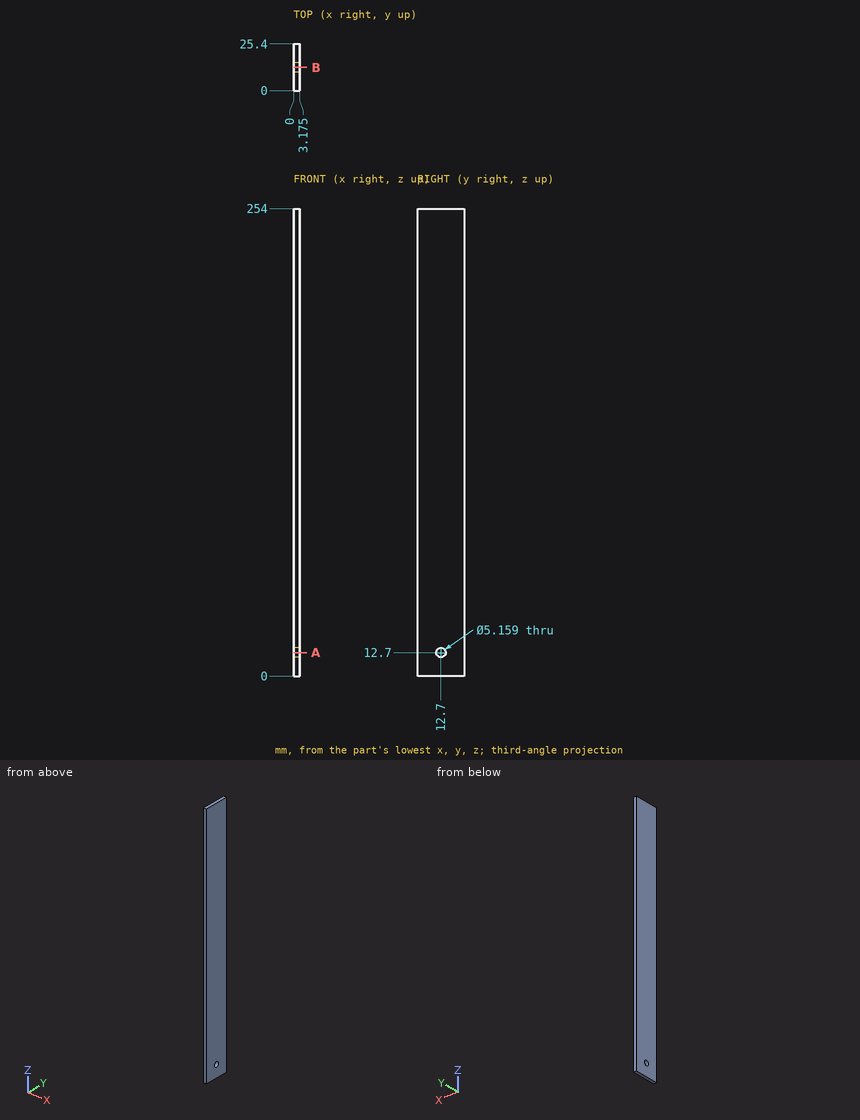
Input: dimensioned drawing with shaded views. Units: mm. Origin: part minimum x, y, z. Coordinates: 2 decimals unless noted, no trailing zeros. Loops run counter-clockwise (first coordinate to the right, second up) from the corner with the lowest first, then second, coordinate; pieces in that order, holes last. Notation, with made-up numbers: (50, 54) - (79, 54) arc R22 ccw to (79, 80) - close; hole circle Ø10 at (44.5, 18). An arc over 180 degrees is marked (long way). One line per question, with ' | ' between items. Start each with the question number.
(1) Cut plane A-A on z = 12.7. Output: boundary loops of the cut face in (x, y) (1 decimal).
(2) Ray query, L1, parallel to Y at x = 2.4, z = 12.7; L2, parallel to Z at x = 1.4, y = 12.7; L3, parallel to Z at x = 1.25, y = 13.5. Return the intervals inside material, ascending. Write a range as from..to.
(3) Cut plane B-B on y = 12.7. Output: boundary loops of the cut face in (x, z) (1 decimal).
Here are the results:
1) outline: (0, 0) - (3.2, 0) - (3.2, 10.1) - (0, 10.1) - close; (0, 15.3) - (3.2, 15.3) - (3.2, 25.4) - (0, 25.4) - close
2) L1: 0..10.12, 15.28..25.4 | L2: 0..10.12, 15.28..254 | L3: 0..10.25, 15.15..254
3) outline: (0, 0) - (3.2, 0) - (3.2, 10.1) - (0, 10.1) - close; (0, 15.3) - (3.2, 15.3) - (3.2, 254) - (0, 254) - close
